Design review of the part built by this model. Coordinates are the model's own, in mm. A direction names the side the tool comes from. Coordinates: 2 decimals unless noted, no trailing zeros. Write each loop counter-clockwise with the first axis right and the second up, starting at its lowest first coordinate (ties: lowest second). Pieces come first, ordered by that corner, then holes.
Q1. For pin 1 Ø3 at (y, z) = (-174.5, 17) entering from -X; pin 2 Ø6 at (y, z) = (172, 5) entering from -X; pin 3 Ø5 at (y, z) = (-155.5, 2) entering from -X; pin 4 Ø12 at (x, y) = (62, 96.5) entering from +Z, all flat-tipped, find the tip position at first contact; note any pin that passes through.
Q2. For faces 5 (the flat face through (-1, -300, 10)), 6 (the flat face through (-1.11, -43.96, 9.86)), list the 3-axis set-ups (+Z, -Z, +X, -X, +Y, -Y) from which the entire face can be reached by the end or side of a thin tool; tool diameter is ignored.
Q3. Take a section at B-B, the plane x = -23.5. Write out the cut boundary in (y, z), plus the area to 3 significant figures.
Q4. Take a section at C-C, the plane z = 11.25. Write out the cut boundary in (x, y), plus the area to 3 significant figures.
Q5. Take a section at D-D, the plane y = 260.5. Write out the cut boundary in (x, z), plus the area to 3 significant figures.
Q6. The part is to be moulded in two halves that separate along Y. For faces 1 (the flat face through (-22, -62, 20)), 2 (the cylindrical face through (58.8, 169.58, 10.14)), 3 (the flat face through (-22.63, 5.28, 9.86)), 4 (the flat face through (67.442, -40, 10)), say which applies: released by +Y, released by -Y, zero draft, split by the parting line, or undercut.
Q7. Take a section at A-A, the plane y = -186.5. Write out the cut boundary in (x, z), plus the area to 3 significant figures.
Q8. For L1, parallel to X at y = -240.5, z = 12.75; L2, parallel to X at y = -201, z = 3.25; L3, parallel to Y at x = 66, z = 14.5, list the stretches that pass through material, from the lowest coordinate up.
from build123d import *

# Parameters (mm, degrees)
F1_DEPTH = 20
F2_R     = 5
F3_R     = 10


with BuildPart() as f1:
    # F0 (on Top) → F1 (new body)
    with BuildSketch(Plane.XY):
        Polygon((95, 300), (47.234748, 300), (-95, -300), (95, -300), align=None)
        Polygon((67.441747, -250.368297), (-50.0391, -250.368297), (67.441747, 245.210379), align=None, mode=Mode.SUBTRACT)
    extrude(amount=F1_DEPTH)

    # F2
    f2_edges = [f1.edges().sort_by_distance(p)[0] for p in [
        (95, 300, 10),
        (95, -300, 10),
        (-95, -300, 10),
        (67.441747, -250.368297, 10),
        (-50.0391, -250.368297, 10),
        (47.234748, 300, 10),
    ]]
    fillet(f2_edges, radius=F2_R)

    # F3
    f3_edges = [f1.edges().sort_by_distance(p)[0] for p in [
        (67.441747, 245.210379, 10),
    ]]
    fillet(f3_edges, radius=F3_R)


solid = f1.part
Responses:
1. pin 1: stops at x = -65.6
1. pin 2: stops at x = 16.18
1. pin 3: stops at x = -61.34
1. pin 4: stops at z = 20
2. face 5: +Z, -Z, +X, -X, -Y
2. face 6: +Z, -Z
3. outline: (-300, 0) - (-250.37, 0) - (-250.37, 20) - (-300, 20) - close; (-138.42, 0) - (1.61, 0) - (1.61, 20) - (-138.42, 20) - close
3. area: 3,790 mm2
4. outline: (-93.54, -293.85) arc R5 ccw to (-88.68, -300) - (90, -300) arc R5 ccw to (95, -295) - (95, 295) arc R5 ccw to (90, 300) - (51.19, 300) arc R5 ccw to (46.32, 296.15) - close; hole (-48.58, -244.21) arc R5 ccw to (-43.72, -250.37) - (62.44, -250.37) arc R5 ccw to (67.44, -245.37) - (67.44, 159.67) arc R10 ccw to (47.71, 161.98) - close
4. area: 42,900 mm2
5. outline: (37.87, 0) - (95, 0) - (95, 20) - (37.87, 20) - close
5. area: 1,140 mm2
6. face 1: zero draft
6. face 2: undercut
6. face 3: released by +Y
6. face 4: undercut
7. outline: (-68.09, 0) - (-34.9, 0) - (-34.9, 20) - (-68.09, 20) - close; (67.44, 0) - (95, 0) - (95, 20) - (67.44, 20) - close
7. area: 1,220 mm2
8. L1: x = -80.9 to -47.7, 67.44 to 95
8. L2: x = -71.53 to -38.34, 67.44 to 95
8. L3: y = -300 to -248.88, 164.85 to 300
